Could you check a few things on this model? Use its own coordinates, in mm. Face numbers are marked on the shaded views. A direction names the side the tool comes from. Round coordinates to 2 decimals unless told otherwise and drop trailing zeros. Write each loop counter-clockwise with the first axis right and the second up, starting at its lowest first coordinate (ties: lowest second). Pieces come first, ordered by that corner, then holes. Notation, with made-up numbers: (34, -29.75) -> (38, -29.75) arc R27 ccw to (38, -5.75) -> close; hole circle Ø9 at (52.25, -0.75). An arc over 180 degrees is marked (long way). Answer in a Markdown table with one row per item.
from build123d import *

# Parameters (mm, degrees)
F0_W      = 5
F0_H      = 95
F0_W_2    = 95
F0_H_2    = 5
F1_DEPTH  = 1.5
F2_R      = 2.75
F2_R_2    = 5
F3_DEPTH  = 1.501
F4_R      = 5
F6_W      = 95
F6_H      = 31
F6_R      = 2.75
F7_DEPTH  = 1.5
F9_W      = 95
F9_H      = 30
F9_R      = 2.7
F10_DEPTH = 1.5
F11_R     = 5
F12_R     = 3.5
F13_R     = 5
F14_SIZE  = 0.4
F15_SIZE  = 0.4


with BuildPart() as f1:
    # F0 (on Top) → F1 (new body)
    with BuildSketch(Plane.XY):
        Polygon((70, 70), (-70, 70), (-70, -70), (-47.5, -70), (47.5, -70), (70, -70), (70, -47.5), (70, 47.5), align=None)
        with Locations((72.5, 0)):
            Rectangle(F0_W, F0_H)
        with Locations((0, -72.5)):
            Rectangle(F0_W_2, F0_H_2)
    extrude(amount=F1_DEPTH)

    # F2 (on face) → F3 (cut, through all)
    with BuildSketch(Plane.XY.offset(1.5)):
        with Locations((-33.5875721064, -33.5875721064)):
            Circle(F2_R)
        with Locations((33.5875721064, -33.5875721064)):
            Circle(F2_R)
        with Locations((-33.5875721064, 33.5875721064)):
            Circle(F2_R)
        with Locations((33.5875721064, 33.5875721064)):
            Circle(F2_R)
        with Locations((0, -33.5875721064)):
            Circle(F2_R_2)
        with Locations((33.5875721064, 0)):
            Circle(F2_R_2)
        with Locations((-33.5875721064, 0)):
            Circle(F2_R_2)
        with Locations((0, 33.5875721064)):
            Circle(F2_R_2)
    extrude(amount=-F3_DEPTH, mode=Mode.SUBTRACT)

    # F4
    f4_edges = [f1.edges().sort_by_distance(p)[0] for p in [
        (70, -70, 0.75),
        (-70, -70, 0.75),
        (70, 70, 0.75),
        (-70, 70, 0.75),
    ]]
    fillet(f4_edges, radius=F4_R)

    # F6 (on 3pt) → F7 (join)
    with BuildSketch(Plane.XZ.offset(75)):
        with Locations((0, -14)):
            Rectangle(F6_W, F6_H)
        with Locations((-40, -15.5)):
            Circle(F6_R, mode=Mode.SUBTRACT)
        with Locations((40, -15.5)):
            Circle(F6_R, mode=Mode.SUBTRACT)
    extrude(amount=-F7_DEPTH)

    # F9 (on 3pt) → F10 (join)
    with BuildSketch(Plane(origin=(75, 0, 0), x_dir=(0, -1, 0), z_dir=(-1, 0, 0))):
        with Locations((0, -13.5)):
            Rectangle(F9_W, F9_H)
        with Locations((-40, -15.5)):
            Circle(F9_R, mode=Mode.SUBTRACT)
        with Locations((40, -15.5)):
            Circle(F9_R, mode=Mode.SUBTRACT)
    extrude(amount=F10_DEPTH)

    # F11
    f11_edges = [f1.edges().sort_by_distance(p)[0] for p in [
        (75, 0, 1.5),
        (0, -75, 1.5),
    ]]
    fillet(f11_edges, radius=F11_R)

    # F12
    f12_edges = [f1.edges().sort_by_distance(p)[0] for p in [
        (73.5, 0, 0),
        (0, -73.5, 0),
    ]]
    fillet(f12_edges, radius=F12_R)

    # F13
    f13_edges = [f1.edges().sort_by_distance(p)[0] for p in [
        (74.25, -47.5, -28.5),
        (47.5, -74.25, -29.5),
        (74.25, 47.5, -28.5),
        (-47.5, -74.25, -29.5),
    ]]
    fillet(f13_edges, radius=F13_R)

    # F14
    f14_edges = [f1.edges().sort_by_distance(p)[0] for p in [
        (-5, -33.587572, 1.5),
        (5, -33.587572, 0.75),
        (-5, -33.587572, 0),
        (-38.587572, 0, 1.5),
        (-28.587572, 0, 0.75),
        (-38.587572, 0, 0),
        (-36.337572, -33.587572, 1.5),
        (-30.837572, -33.587572, 0.75),
        (-36.337572, -33.587572, 0),
        (30.837572, -33.587572, 1.5),
        (36.337572, -33.587572, 0.75),
        (30.837572, -33.587572, 0),
        (28.587572, 0, 1.5),
        (38.587572, 0, 0.75),
        (28.587572, 0, 0),
        (-5, 33.587572, 1.5),
        (5, 33.587572, 0.75),
        (-5, 33.587572, 0),
        (-36.337572, 33.587572, 1.5),
        (-30.837572, 33.587572, 0.75),
        (-36.337572, 33.587572, 0),
        (30.837572, 33.587572, 1.5),
        (36.337572, 33.587572, 0.75),
        (30.837572, 33.587572, 0),
    ]]
    chamfer(f14_edges, length=F14_SIZE)

    # F15
    f15_edges = [f1.edges().sort_by_distance(p)[0] for p in [
        (42.75, -74.25, -15.5),
        (37.25, -75, -15.5),
        (37.25, -73.5, -15.5),
        (-37.25, -74.25, -15.5),
        (-42.75, -75, -15.5),
        (-42.75, -73.5, -15.5),
        (74.25, -42.7, -15.5),
        (75, -37.3, -15.5),
        (73.5, -37.3, -15.5),
        (74.25, 37.3, -15.5),
        (75, 42.7, -15.5),
        (73.5, 42.7, -15.5),
    ]]
    chamfer(f15_edges, length=F15_SIZE)


solid = f1.part
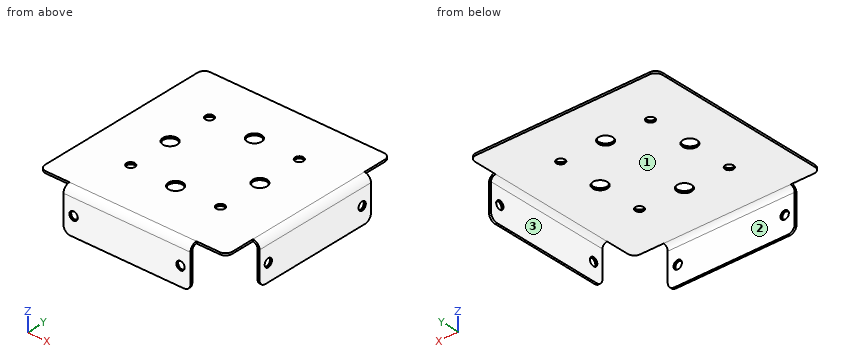
1) Imagine slicing it at D-D, the plane z = -15.5. Count the separate pieces of the cut face and the enclosed holes in it, plus the area to 3 significant figures.
Findings:
| item | result |
|---|---|
| separate pieces | 6 |
| enclosed holes | 0 |
| area | 251 mm^2 |
2) Imagine slicing it at A-A, the plane z = -6. Please give me the cut outline in (x, y).
Findings:
| item | result |
|---|---|
| outline | (-47.5, -75) -> (47.5, -75) -> (47.5, -73.5) -> (-47.5, -73.5) -> close; (73.5, -47.5) -> (75, -47.5) -> (75, 47.5) -> (73.5, 47.5) -> close |
3) Imagine slicing it at B-B, the plane x = 0. Please give me the cut outline in (y, z).
Findings:
| item | result |
|---|---|
| outline | (-75, -29.5) -> (-73.5, -29.5) -> (-73.5, -3.5) arc R3.5 cw to (-70, 0) -> (-38.99, 0) -> (-38.59, 0.4) -> (-38.59, 1.1) -> (-38.99, 1.5) -> (-70, 1.5) arc R5 ccw to (-75, -3.5) -> close; (-28.59, 0.4) -> (-28.19, 0) -> (28.19, 0) -> (28.59, 0.4) -> (28.59, 1.1) -> (28.19, 1.5) -> (-28.19, 1.5) -> (-28.59, 1.1) -> close; (38.59, 0.4) -> (38.99, 0) -> (70, 0) -> (70, 1.5) -> (38.99, 1.5) -> (38.59, 1.1) -> close |
4) Please list where these lines run through material, in increasing order: line 1 (Y direction, x = -37.5, z = -4); line 2 (Z direction, x = -60, y = 26); line 3 (X direction, y = 11, z = -21.5).
Findings:
| item | result |
|---|---|
| line 1 | y = -75 to -73.5 |
| line 2 | z = 0 to 1.5 |
| line 3 | x = 73.5 to 75 |
5) For the marked faces 1, 2 and 3, which set-ups out of +Z, -Z, +X, -X, +Y, -Y let a thin tool reach every point of the face, with its end or its side?
Findings:
| item | result |
|---|---|
| face 1 | -Z, -X, +Y |
| face 2 | -Z, +X, -X, +Y |
| face 3 | -Z, -X, +Y, -Y |
6) For pin 1 (8 mm diameter, centred on x = 33.59, y = 0, fed in from +Z); pin 2 (4 mm diameter, centred on x = -34.5, y = -39, fed in from -Z); pin 3 (4 mm diameter, centred on y = -73.5, z = -13.5, fed in from +X); pin 4 (0.8 mm diameter, centred on x = 74, y = -16.5, fed in from -Z), each with a flat end and sliding along its axis, tell me the tip position at first contact or that it passes through.
Findings:
| item | result |
|---|---|
| pin 1 | passes through |
| pin 2 | stops at z = 0 |
| pin 3 | stops at x = 47.5 |
| pin 4 | stops at z = -28.5 |
7) Imagine slicing it at C-C, the plane y = -16. Please give me the cut outline in (x, z).
Findings:
| item | result |
|---|---|
| outline | (-70, 0) -> (70, 0) arc R3.5 cw to (73.5, -3.5) -> (73.5, -28.5) -> (75, -28.5) -> (75, -3.5) arc R5 ccw to (70, 1.5) -> (-70, 1.5) -> close |
